Build history of the part. All positions in model axes, mm. A direction names the side the tool comes from. Give positions to 0.01 mm unless a question says otherwise; leave off trailing zeros. Loops run counter-clockwise (first coordinate to the right, second up) from the corner with the lowest first, then second, coordinate; pieces in that order, holes last.
1) Two-plate mould, pull along X, no slides. Class faces 1 (the flat face through (0, 3, -2)), 2 (the flat face through (12, 3, -4)), 3 (the flat face through (5.86, 6.73, -1.97)): +X half, -X half, draft (parallel to the pull), parting line (faces both ways), or undercut.
2) Flat gauge pin, fed straight in: P1, Ø2, axis at x = 15.5, z = -1, coming from the -Y side. Where does the tip first touch, or does it go through?
3) Wall check: line 1 (X direction, y = 2, z = -2.6); line 2 (Y direction, x = 14, z = -2.6) (3 decimals); line 3 (X direction, y = 2.75, z = -2.5). Give the ranges that are in metal, low to high.
4) Band-saw the part on C-C on y = -0.75. List the corners of the cut face in (x, z).
5) Band-saw the part on A-A on y = 3.25. List the corners of the cut face in (x, z), then the cut area to 3 significant figures.
6) 3-axis set-ups, long thin cutter, end or side, ignore diameter. For faces 4 (the flat face through (12, 0, -1)), 5 (the flat face through (12.3, -2, -3.4)), 6 (the flat face through (12.142, 6.73, -1.972)): which of +Z, -Z, +X, -X, +Y, -Y reach the whole face in a straight line?
7) Band-saw the part on B-B on z = -1.85. State how many separate pieces and enclosed holes the cut face has, then the cut area to 3 significant figures.
```python
from build123d import *

# Parameters (mm, degrees)
BLANKSKE_W          = 25
BLANKSKE_H          = 7.3
BLANK_DEPTH         = 4
TOOTHCUTSIM_DEPTH   = 27.349383294
TEETHCUTS_COUNT     = 17
TEETHCUTS_PITCH     = 1.570796325
CUT_EXTRUDE1_DEPTH  = 27.349383294
SKETCH4_W           = 25
SKETCH4_H           = 1.13
BOSS_EXTRUDE1_DEPTH = 2


with BuildPart() as part:
    # BlankSke → Blank (new body)
    with BuildSketch(Plane.XY):
        with Locations((12.5, 3.65)):
            Rectangle(BLANKSKE_W, BLANKSKE_H)
    extrude(amount=-BLANK_DEPTH)

    # TooCutSkeSim → ToothCutSim (cut, through all)
    with BuildSketch(Plane.XY):
        Polygon((0.222217685, 6.175), (-0.222217685, 6.175), (-0.640929042, 7.3254), (0.640929042, 7.3254), align=None)
    toothcutsim = extrude(amount=-TOOTHCUTSIM_DEPTH, mode=Mode.SUBTRACT)

    # TeethCuts: ToothCutSim ×17
    with Locations(*[(i * TEETHCUTS_PITCH, 0, 0) for i in range(1, TEETHCUTS_COUNT)]):
        add(toothcutsim, mode=Mode.SUBTRACT)

    # Sketch1 → Cut-Extrude1 (cut, through all)
    with BuildSketch(Plane(origin=(0, 0, -4), x_dir=(-1, 0, 0), z_dir=(0, 0, -1))):
        with BuildLine():
            Line((-23, 1), (-23, 2))
            Line((-23, 2), (-24, 2))
            ThreePointArc((-24, 2), (-23.707106781, 1.292893219), (-23, 1))
        make_face()
        with BuildLine():
            Line((-24, 2), (-23, 2))
            Line((-23, 2), (-23, 3))
            ThreePointArc((-23, 3), (-23.707106781, 2.707106781), (-24, 2))
        make_face()
        with BuildLine():
            Line((-23, 3), (-23, 2))
            Line((-23, 2), (-23, 1))
            ThreePointArc((-23, 1), (-22.292893219, 1.292893219), (-22, 2))
            ThreePointArc((-22, 2), (-22.292893219, 2.707106781), (-23, 3))
        make_face()
        with BuildLine():
            ThreePointArc((-17, 2), (-18.5, 3.5), (-20, 2))
            Line((-20, 2), (-17, 2))
        make_face()
        with BuildLine():
            Line((-17, 2), (-20, 2))
            ThreePointArc((-20, 2), (-18.5, 0.5), (-17, 2))
        make_face()
        with BuildLine():
            ThreePointArc((-13, 2), (-14, 3), (-15, 2))
            Line((-15, 2), (-13, 2))
        make_face()
        with BuildLine():
            Line((-13, 2), (-15, 2))
            ThreePointArc((-15, 2), (-14, 1), (-13, 2))
        make_face()
        with BuildLine():
            ThreePointArc((-3, 2), (-4, 3), (-5, 2))
            Line((-5, 2), (-3, 2))
        make_face()
        with BuildLine():
            Line((-3, 2), (-5, 2))
            ThreePointArc((-5, 2), (-4, 1), (-3, 2))
        make_face()
    extrude(amount=-CUT_EXTRUDE1_DEPTH, mode=Mode.SUBTRACT)

    # Sketch4 → Boss-Extrude1 (add)
    with BuildSketch(Plane.XZ):
        with Locations((12.5, -3.435)):
            Rectangle(SKETCH4_W, SKETCH4_H)
    extrude(amount=BOSS_EXTRUDE1_DEPTH)


solid = part.part
```
Findings below:
1. face 1: -X half
1. face 2: draft
1. face 3: undercut
2. P1: stops at y = 0
3. line 1: x = 0 to 3, 5 to 13, 15 to 17, 20 to 22, 24 to 25
3. line 2: y = 0 to 1, 3 to 6.175
3. line 3: x = 0 to 3.34, 4.66 to 13.34, 14.66 to 17.2, 19.8 to 22.34, 23.66 to 25
4. outline: (0, -4) - (25, -4) - (25, -2.87) - (0, -2.87) - close
5. outline: (0, -4) - (17.67, -4) - (17.67, 0) - (0, 0) - close; (19.33, -4) - (25, -4) - (25, 0) - (19.33, 0) - close
5. area: 93.4 mm2
6. face 4: +Z, +X, -X, -Y
6. face 5: +Z, -Z, +X, -X, -Y
6. face 6: +Z, -Z, +Y
7. separate pieces: 1
7. enclosed holes: 4
7. area: 151 mm2
